Geometry check sheet. Reference: the model listing, model coordinates, mm. Face numbers are marked on the shaded views. A direction names the side the tool comes from. Round coordinates to 2 decimals unless told otherwise and drop trailing zeros. Order: outer loops, then holes, each group sorted by start corner. A loop starts at its lowest first (then second) coordinate and runs counter-clockwise, first axis right, second up. Notation, with made-up numbers: (-23, -32.75) - (2, -32.75) arc R5 cw to (2, -26.75) - close; hole circle Ø9 at (77, 53). An arc over 180 degrees is marked (long way). Return JSON: item names as keys, results as strings. Group by question number.
Q1. Material ranges on line 1 along X through (y, z) = (0, 30); line 2 along Z through (x, y) = (-34.5, 11), recorded low to high.
Q2. Sectioned sample at A-A, the plane z = 27. Record the cut outline in (x, y), then the cut area to 3 significant figures.
Q3. Gauge pin test, flat ends, axial feed: pin 1 Ø4 at (x, z) = (10.5, 12) entering from -Y; pin 2 Ø18.5 at (y, z) = (-5, 11) entering from -X; pin 3 Ø18.5 at (x, z) = (5.5, 15.5) entering from +Y; pin 4 Ø25 at (x, y) = (5, -11) entering from -Z. Record the tip position at first contact, or that the pin passes through.
Q4. Draft check along X on the marked faces 4, 5 and 6. Enter one of: pulls with the +X half, pulls with the -X half, needs draft (parallel to the pull), parting line crosses it, or undercut.
Q5. Tool access check on the marked faces 1, 2 and 3. Record the directions out of +Z, -Z, +X, -X, +Y, -Y that give a thin tool (end or side, any length) a straight path to the whole face; none if there is none.
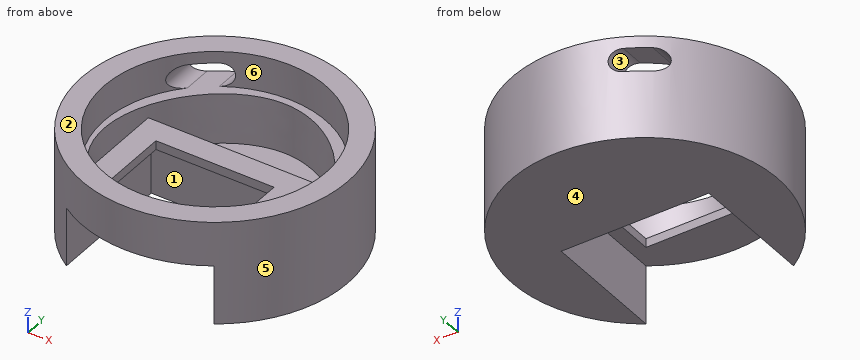
```python
from build123d import *

# Parameters (mm, degrees)
CYLINDER_R      = 45
CYLINDER_DEPTH  = 35
SKETCH_R        = 37.5
POCKET_DEPTH    = 12
SKETCH001_W     = 50
SKETCH001_H     = 75
POCKET001_DEPTH = 20
SKETCH002_W     = 40
SKETCH002_H     = 30
POCKET002_DEPTH = 5
POCKET003_DEPTH = 17
POCKET004_DEPTH = 50


with BuildPart() as part:
    # Cylinder → Cylinder (join)
    with BuildSketch(Plane.XY):
        Circle(CYLINDER_R)
    extrude(amount=CYLINDER_DEPTH)

    # Sketch (on Face3 of Cylinder) → Pocket (cut)
    with BuildSketch(Plane.XY.offset(35)):
        Circle(SKETCH_R)
    extrude(amount=-POCKET_DEPTH, mode=Mode.SUBTRACT)

    # Sketch001 (on Face2 of Pocket) → Pocket001 (cut)
    with BuildSketch(Plane(origin=(0, 0, 0), x_dir=(1, 0, 0), z_dir=(0, 0, -1))):
        with Locations((0, 32.5)):
            Rectangle(SKETCH001_W, SKETCH001_H)
    extrude(amount=-POCKET001_DEPTH, mode=Mode.SUBTRACT)

    # Sketch002 (on Face4 of Pocket001) → Pocket002 (cut)
    with BuildSketch(Plane(origin=(0, 0, 20), x_dir=(1, 0, 0), z_dir=(0, 0, -1))):
        with Locations((0, 15)):
            Rectangle(SKETCH002_W, SKETCH002_H)
    extrude(amount=-POCKET002_DEPTH, mode=Mode.SUBTRACT)

    # Sketch003 (on Face13 of Pocket002) → Pocket003 (cut)
    with BuildSketch(Plane.XY.offset(23)):
        with BuildLine():
            Line((28, -22), (28, 8))
            Line((28, 8), (-28, 8))
            Line((-28, 8), (-28, -22))
            add(Edge.make_bspline(
                [(-28, -22), (-48, 0), (0, 70), (48, 0), (28, -22)],
                knots=[0, 0, 0, 0, 0.5, 1, 1, 1, 1], degree=3))
        make_face()
    extrude(amount=-POCKET003_DEPTH, mode=Mode.SUBTRACT)

    # Sketch004 (on DatumPlane) → Pocket004 (cut)
    with BuildSketch(Plane.XZ.offset(-5)):
        with BuildLine():
            ThreePointArc((-27, 31), (-31, 27), (-27, 23))
            Line((-27, 23), (-20, 23))
            ThreePointArc((-20, 23), (-16, 27), (-20, 31))
            Line((-20, 31), (-27, 31))
        make_face()
    extrude(amount=-POCKET004_DEPTH, mode=Mode.SUBTRACT)


solid = part.part
```
Reply:
{
 "1": {"line 1": "-45 to -37.5, 37.5 to 45", "line 2": "0 to 23"},
 "2": {"outline": "(-31, 21.1) - (-31, 32.62) arc R45 ccw (long way) to (-16, 42.06) - (-16, 33.92) arc R37.5 cw (long way) to start", "area": "1,800 mm^2"},
 "3": {"pin 1": "y = 5", "pin 2": "x = -45", "pin 3": "y = 45", "pin 4": "z = 20"},
 "4": {"face 4": "needs draft", "face 5": "parting line crosses it", "face 6": "undercut"},
 "5": {"face 1": "-Z, -Y", "face 2": "+Z, +X, -X, +Y, -Y", "face 3": "+Y"}
}
